Verification items for this drawing (mm, ordinates from the low corner). A direction names the side the tool comes from. Round coordinates to 2 decimals unless told otherwise and drop trailing zeros. Loops run counter-clockwise (first coordinate to the right, second up) from the corner with the lowest first, then second, coordinate; pieces in that order, holes last. Notation, with made-up numbers: M 61.25,68.5 L 85.25,68.5 A14 cw 85.25,86.5 Z; hole C 18.25,-23.75 d9. An arc over 180 degrees is marked long. Write item = value, one per line. Start each with the question number.
(1) Cross-section at C-C on z = 18. Record the boundary of the cut face in (x, y), plus the area to 3 significant figures.
(2) Set-up check for the marked faces 1 and 2: record each of +Z, -Z, +X, -X, +Y, -Y from which the full face is reachable in a straight line by a thin tool's end or side.
(3) Scan lines: L1, parallel to Z at x = 10.5, y = 5.25; L2, parallel to Y at x = 4, z = 21. Record each from-to range of solid material in increasing order. Write a range as from..to.
(4) Go/stop test with flat-tipped pins: P1, Ø8.5, axis at x = 9.5, y = 3, coming from the +Z side; P2, Ø4, axis at x = 9.5, z = 26.5, coming from the -Y side. Record where each tip stops, or that it passes through.
(5) Cross-section at B-B on x = 14.75. Record the boundary of the cut face in (y, z) (1 decimal).
(6) Cross-section at A-A on y = 2.25. Record the boundary of the cut face in (x, z), plus the area to 3 significant figures.
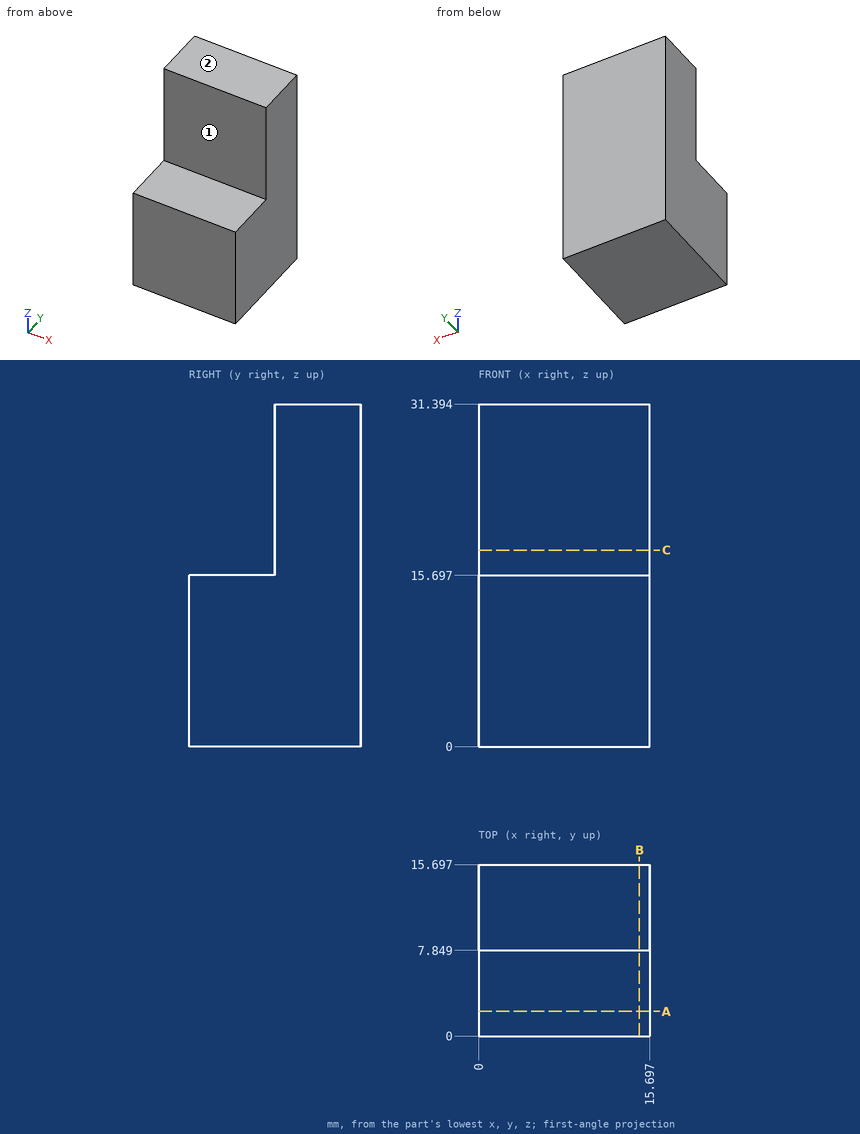
Result:
q1.outline = M 0,7.85 L 15.7,7.85 L 15.7,15.7 L 0,15.7 Z
q1.area = 123 mm^2
q2.face_1 = +Z, +X, -X, -Y
q2.face_2 = +Z, +X, -X, +Y, -Y
q3.L1 = 0..15.7
q3.L2 = 7.85..15.7
q4.P1 = 15.7
q4.P2 = 7.85
q5.outline = M 0,0 L 15.7,0 L 15.7,31.4 L 7.8,31.4 L 7.8,15.7 L 0,15.7 Z
q6.outline = M 0,0 L 15.7,0 L 15.7,15.7 L 0,15.7 Z
q6.area = 246 mm^2
